```python
from build123d import *

# Parameters (mm, degrees)
SKETCH_1_R          = 1.6
SKETCH_1_R_2        = 5.05
EXTRUDE_1_DEPTH     = 3
SKETCH_2_R          = 1.6
CUT_EXTRUDE_1_DEPTH = 124.535581919
SKETCH_3_R          = 1.6
CUT_EXTRUDE_2_DEPTH = 124.535581919
FILLET_1_R          = 1
EXTRUDE_START       = -3
EXTRUDE_2_DEPTH     = 3
CHAMFER_1_SIZE      = 1.75
CHAMFER_2_SIZE      = 1.75


with BuildPart() as part:
    # ｽｹｯﾁ1 → ﾎﾞｽ - 押し出し1 (new body)
    with BuildSketch(Plane.XY):
        with BuildLine():
            Line((-2.227171492, 19.875605831), (86.459242762, 29.813408746))
            ThreePointArc((86.459242762, 29.813408746), (119.8, 0), (86.459242762, -29.813408746))
            Line((86.459242762, -29.813408746), (-2.227171492, -19.875605831))
            ThreePointArc((-2.227171492, -19.875605831), (-20, 0), (-2.227171492, 19.875605831))
        make_face()
        Circle(SKETCH_1_R, mode=Mode.SUBTRACT)
        with Locations((89.8, 0)):
            Circle(SKETCH_1_R_2, mode=Mode.SUBTRACT)
    extrude(amount=EXTRUDE_1_DEPTH)

    # ｽｹｯﾁ2 → ｶｯﾄ - 押し出し1 (cut, through all)
    with BuildSketch(Plane.XY.offset(3)):
        with Locations((89.8, 10)):
            Circle(SKETCH_2_R)
        with Locations((99.8, 0)):
            Circle(SKETCH_2_R)
        with Locations((89.8, -10)):
            Circle(SKETCH_2_R)
        with Locations((79.8, 0)):
            Circle(SKETCH_2_R)
    extrude(amount=-CUT_EXTRUDE_1_DEPTH, mode=Mode.SUBTRACT)

    # ｽｹｯﾁ3 → ｶｯﾄ - 押し出し2 (cut, through all)
    with BuildSketch(Plane.XY.offset(3)):
        with Locations((21.127828075, 17.209804787)):
            Circle(SKETCH_3_R)
        with Locations((21.127828075, -17.209804787)):
            Circle(SKETCH_3_R)
        with Locations((60.046685431, -21.570877871)):
            Circle(SKETCH_3_R)
        with Locations((60.046685431, 21.570877871)):
            Circle(SKETCH_3_R)
        Polygon((24.311632117, 17.566567628), (56.056085363, 21.123709076), (38.398951009, 3.529263334), align=None)
        Polygon((24.311632117, -17.566567628), (56.056085363, -21.123709076), (38.398951009, -3.529263334), align=None)
        with BuildLine():
            Line((22.640031329, 12.173707016), (34.857112989, 0))
            Line((34.857112989, 0), (22.640031329, -12.173707016))
            ThreePointArc((22.640031329, -12.173707016), (21.34147622, -12.270762122), (21.047953505, -11.002097675))
            ThreePointArc((21.047953505, -11.002097675), (23.75, 0), (21.047953505, 11.002097675))
            ThreePointArc((21.047953505, 11.002097675), (21.34147622, 12.270762122), (22.640031329, 12.173707016))
        make_face()
        with BuildLine():
            Line((58.927113914, 16.926017866), (41.940789029, 0))
            Line((41.940789029, 0), (58.927113914, -16.926017866))
            ThreePointArc((58.927113914, -16.926017866), (60.230336409, -17.019617306), (60.513751544, -15.744146574))
            ThreePointArc((60.513751544, -15.744146574), (56.55, 0), (60.513751544, 15.744146574))
            ThreePointArc((60.513751544, 15.744146574), (60.230336409, 17.019617306), (58.927113914, 16.926017866))
        make_face()
    extrude(amount=-CUT_EXTRUDE_2_DEPTH, mode=Mode.SUBTRACT)

    # ﾌｨﾚｯﾄ1
    fillet_1_edges = [part.edges().sort_by_distance(p)[0] for p in [
        (56.056085363, 21.123709076, 1.5),
        (38.398951009, 3.529263334, 1.5),
        (24.311632117, 17.566567628, 1.5),
        (41.940789029, 0, 1.5),
        (24.311632117, -17.566567628, 1.5),
        (38.398951009, -3.529263334, 1.5),
        (56.056085363, -21.123709076, 1.5),
        (34.857112989, 0, 1.5),
    ]]
    fillet(fillet_1_edges, radius=FILLET_1_R)

    # ｽｹｯﾁ4 → ﾎﾞｽ - 押し出し2 (add)
    with BuildSketch(Plane.XY.offset(3).offset(EXTRUDE_START)):
        with BuildLine():
            Line((81.98967358, 30.426942029), (1.294053754, 21.796225015))
            ThreePointArc((1.294053754, 21.796225015), (-8.232619041, 18.767269305), (-15.81095889, 12.248003061))
            ThreePointArc((-15.81095889, 12.248003061), (-9.792273379, 17.438789582), (-2.227171492, 19.875605831))
            Line((-2.227171492, 19.875605831), (86.459242762, 29.813408746))
            ThreePointArc((86.459242762, 29.813408746), (93.570181832, 29.762152626), (100.46928661, 28.038657657))
            ThreePointArc((100.46928661, 28.038657657), (91.370486749, 30.323854341), (81.98967358, 30.426942029))
        make_face()
        with BuildLine():
            ThreePointArc((-2.227171492, -19.875605831), (-9.792273379, -17.438789582), (-15.81095889, -12.248003061))
            ThreePointArc((-15.81095889, -12.248003061), (-8.232619041, -18.767269305), (1.294053754, -21.796225015))
            Line((1.294053754, -21.796225015), (81.98967358, -30.426942029))
            ThreePointArc((81.98967358, -30.426942029), (91.370486749, -30.323854341), (100.46928661, -28.038657657))
            ThreePointArc((100.46928661, -28.038657657), (93.570181832, -29.762152626), (86.459242762, -29.813408746))
            Line((86.459242762, -29.813408746), (-2.227171492, -19.875605831))
        make_face()
    extrude(amount=EXTRUDE_2_DEPTH)

    # 面取り1
    chamfer_1_edges = [part.edges().sort_by_distance(p)[0] for p in [
        (-1.6, 0, 0),
        (19.527828075, -17.209804787, 0),
        (58.446685431, -21.570877871, 0),
        (58.446685431, 21.570877871, 0),
        (19.527828075, 17.209804787, 0),
    ]]
    chamfer(chamfer_1_edges, length=CHAMFER_1_SIZE)

    # 面取り2
    chamfer_2_edges = [part.edges().sort_by_distance(p)[0] for p in [
        (88.2, 10, 3),
        (98.2, 0, 3),
        (88.2, -10, 3),
        (78.2, 0, 3),
    ]]
    chamfer(chamfer_2_edges, length=CHAMFER_2_SIZE)


solid = part.part
```
Verification items for the finished model (mm, model axes). A direction names the side the tool comes from. Round coordinates to 2 decimals unless told otherwise and drop trailing zeros. Order: outer loops, then holes, each group sorted by start corner. A loop starts at its lowest first (then second) coordinate and runs counter-clockwise, first axis right, second up.
1) Cross-section at D-D, the plane x = 89.8. Record the cut outline in (y, z).
Geometry says:
outline: (-30.5, 0) - (-11.6, 0) - (-11.6, 1.25) - (-13.35, 3) - (-30.5, 3) - close; (-8.4, 0) - (-5.05, 0) - (-5.05, 3) - (-6.65, 3) - (-8.4, 1.25) - close; (5.05, 0) - (8.4, 0) - (8.4, 1.25) - (6.65, 3) - (5.05, 3) - close; (11.6, 0) - (30.5, 0) - (30.5, 3) - (13.35, 3) - (11.6, 1.25) - close
2) Material ranges on line 1 (X direction, y = 7, z = 0.55) (3 decimals); line 2 (X direction, y = 12, z = 0.7); line 3 (Y direction, x = 86, z = 0.95), recorded low to high.
Geometry says:
line 1: x = -18.735 to 22.695, 27.832 to 34.916, 41.882 to 48.966, 57.295 to 118.972
line 2: x = -16 to 21.09, 22.81 to 29.9, 46.9 to 53.98, 58.79 to 117.3
line 3: y = -30.65 to -3.33, 3.33 to 30.65
3) Cross-section at B-B, the plane x = 50. Record the cut outline in (y, z), plus the area to 3 significant figures.
Geometry says:
outline: (-27.01, 0) - (-20.45, 0) - (-20.45, 3) - (-27.01, 3) - close; (-15.09, 0) - (-8.03, 0) - (-8.03, 3) - (-15.09, 3) - close; (8.03, 0) - (15.09, 0) - (15.09, 3) - (8.03, 3) - close; (20.45, 0) - (27.01, 0) - (27.01, 3) - (20.45, 3) - close
area: 81.7 mm2
4) Cross-section at A-A, the plane x = 0. Record the cut outline in (y, z).
Geometry says:
outline: (-21.62, 0) - (-3.35, 0) - (-1.6, 1.75) - (-1.6, 3) - (-21.62, 3) - close; (1.6, 1.75) - (3.35, 0) - (21.62, 0) - (21.62, 3) - (1.6, 3) - close
5) Tool access check on faces 4 (the flat face through (46.7, -11.8, 1.5)), 5 (the flat face through (42.207, 26.172, 1.479)). Record the directions out of +Z, -Z, +X, -X, +Y, -Y that give a thin tool (end or side, any length) a straight path to the whole face; none if there is none.
Geometry says:
face 4: +Z, -Z
face 5: +Z, -Z, -X, +Y
6) Cross-section at C-C, the plane z = 2.2. Give the number of separate pieces and of enclosed holes in the cut face, plus the area to 3 significant figures.
Geometry says:
separate pieces: 1
enclosed holes: 14
area: 5,720 mm2
7) Depth check by flat-ended pin: pin 1 (3.5 mm diameter, centred on x = 60.05, y = 21.57, fed in from -Z); pin 2 (5 mm diameter, centred on x = 21.13, y = 17.21, fed in from -Z); pin 3 (4 mm diameter, centred on x = 89.8, y = -10, fed in from +Z). Enter the tip coordinate at first touch or a pass-through.
Geometry says:
pin 1: stops at z = 1.6
pin 2: stops at z = 0.85
pin 3: stops at z = 1.65
8) Draft check along Y on faces 1 (the flat face through (31.823, -10.081, 1.521)), 2 (the flat face through (48.9, 7.2, 3)), 3 (the cylindrical face through (-8.355, -18.698, 1.479)). Enter one of: +Y half, -Y half, draft (parallel to the pull), parting line (faces both ways), or undercut.
Geometry says:
face 1: undercut
face 2: draft
face 3: -Y half
